from build123d import *

# Parameters (mm, degrees)
BOSS_EXTRUDE2_DEPTH = 3.175
BOSS_EXTRUDE3_DEPTH = 3.175
CUT_EXTRUDE2_DEPTH  = 958.917567573


with BuildPart() as part:
    # Sketch3 → Boss-Extrude2 (new body)
    with BuildSketch(Plane(origin=(0, 0, 0), x_dir=(0, 0, -1), z_dir=(0.9227400229187457, 0.3854229496331436, 0))):
        Polygon((0, 0), (609.6, 0), (628.65, 304.8), (514.35, 643.582154794), (95.25, 643.582154794), (-19.05, 304.8), align=None)
    extrude(amount=BOSS_EXTRUDE2_DEPTH)

    # Sketch4 → Boss-Extrude3 (add)
    with BuildSketch(Plane(origin=(0, 595.08273013, 0), x_dir=(1, 0, 0), z_dir=(0, 1, 0))):
        with BuildLine():
            Line((-245.121632859, 514.35), (-388.214384584, 468.215025945))
            ThreePointArc((-388.214384584, 468.215025945), (-404.136734332, 456.688108103), (-410.221632859, 437.996798187))
            Line((-410.221632859, 437.996798187), (-410.221632859, 171.603201813))
            ThreePointArc((-410.221632859, 171.603201813), (-404.136734332, 152.911891897), (-388.214384584, 141.384974055))
            Line((-388.214384584, 141.384974055), (-245.121632859, 95.25))
            Line((-245.121632859, 95.25), (-245.121632859, 514.35))
        make_face()
    extrude(amount=-BOSS_EXTRUDE3_DEPTH)

    # Sketch5 → Cut-Extrude2 (cut, through all)
    with BuildSketch(Plane(origin=(0, 0, 0), x_dir=(0, 0, -1), z_dir=(0.9227400229187457, 0.3854229496331436, 0))):
        Polygon((609.6, 0), (627.0625, 279.4), (520.7, 0), align=None)
    extrude(amount=CUT_EXTRUDE2_DEPTH, mode=Mode.SUBTRACT)


solid = part.part
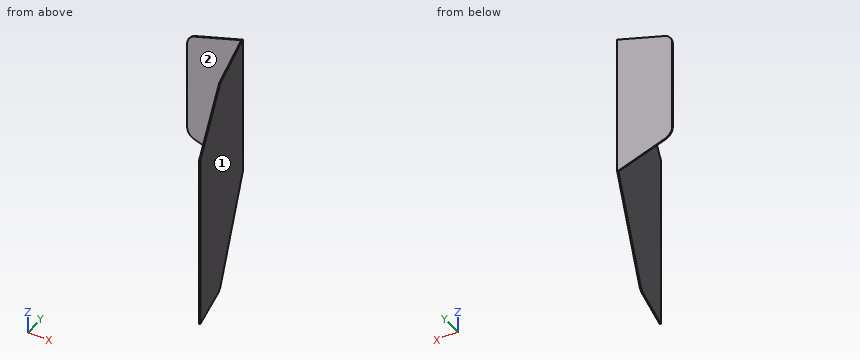
Here's how the part is built. I have some questions about the finished solid (model axes, mm). Face numbers are marked on the shaded views. A direction names the side the tool comes from. Give positions to 0.01 mm unless a question says otherwise; leave off trailing zeros. Order: outer loops, then holes, each group sorted by start corner. A loop starts at its lowest first (then second) coordinate and runs counter-clockwise, first axis right, second up. Notation, with made-up numbers: (-8, 49) -> (22, 49) arc R17 cw to (22, 78) -> close; hole circle Ø7 at (-21, 14). An arc over 180 degrees is marked (long way). Use a Markdown table: item, result. Add a question column.
Item 1: Imagine slicing it at A-A on z = -284.5. Please give me the cut outline in (x, y), plus the area to 3 significant figures.
Item 2: Will these pins go through, and if not, where does the flat tip stop? pin 1 (5 mm diameter, centred on x = -196.5, z = -505.5, fed in from -Y); pin 2 (8 mm diameter, centred on x = -123.5, z = -335.5, fed in from -Y); pin 3 (10 mm diameter, centred on y = 514, z = -358.5, fed in from -X).
Item 3: I need wall thicknesses on line 1 (Y direction, x = -297, z = -116.5); line 2 (X direction, y = 171, z = -22.5); line 3 (X direction, y = 438, z = -566). Which ranges of each line are inside material? Lowest first, please.
Item 4: For the marked faces 1 and 2, which set-ups out of +Z, -Z, +X, -X, +Y, -Y let a thin tool reach every point of the face, with its end or its side?
Item 5: Imagine slicing it at C-C on x = -189. Please give me the cut outline in (y, z), plus the area to 3 significant figures.
Item 6: Imagine slicing it at B-B on y = 390. Please give me the cut outline in (x, z), plus the area to 3 significant figures.
Data:
| question | item | result |
|---|---|---|
| 1 | outline | (-410.22, 591.91) -> (-247.24, 591.91) -> (0, 0) -> (2.93, 1.22) -> (-245.12, 595.08) -> (-410.22, 595.08) -> close |
| 1 | area | 2,560 mm² |
| 2 | pin 1 | stops at y = 464.45 |
| 2 | pin 2 | stops at y = 286.09 |
| 2 | pin 3 | stops at x = -216.78 |
| 3 | line 1 | y = 591.91 to 595.08 |
| 3 | line 2 | x = -71.43 to -67.98 |
| 3 | line 3 | x = -182.95 to -179.51 |
| 4 | face 1 | +Z, -Z, +X, +Y |
| 4 | face 2 | +Z, -Z, -X, -Y |
| 5 | outline | (452.48, -566.04) -> (460.72, -563.48) -> (460.72, -46.12) -> (452.48, -43.56) -> close |
| 5 | area | 4,280 mm² |
| 6 | outline | (-162.9, -588.89) -> (-159.46, -589.34) -> (-159.46, -20.26) -> (-162.9, -20.71) -> close |
| 6 | area | 1,960 mm² |
